The listing builds one solid part. Answer for the finished solid, in the listing's coordinates (mm). Give positions to 0.01 mm unless a question says otherwise; leave off trailing zeros. Order: outer loops, then holes, each group sorted by start corner. A loop starts at its lowest first (then second) coordinate and runs counter-clockwise, first axis right, second up. Notation, with made-up numbers: (-33.75, 8) - (12.25, 8) arc R32 cw to (12.25, 35) - close; hole circle Ø5 at (32.25, 65.5). An arc over 180 degrees is marked (long way). Answer as a JSON object with one key per item and string values. Group by question number.
Q1. A cutting plane is placed at B-B, the plane y = 4. Give the vertices of the cut face in (x, z), and give its area (3 significant figures).
Q2. Consider line 1 (Y direction, x = -5.5, z = 304.5); line 2 (Y direction, x = -13, z = 213.5). Determine where each line is inside the solid, lowest interval first.
Q3. A cutting plane is placed at C-C, the plane z = 54. Give the vertices of the cut face in (x, y).
Q4. A cutting plane is placed at A-A, the plane x = -6. Give the vertices of the cut face in (y, z).
Q5. Given pin 1 (2 mm diameter, centred on x = 6, y = -12.5, fed in from +Z), flat-ended and moving along its own axis, determine where the tip first touches the part or whether it passes through.
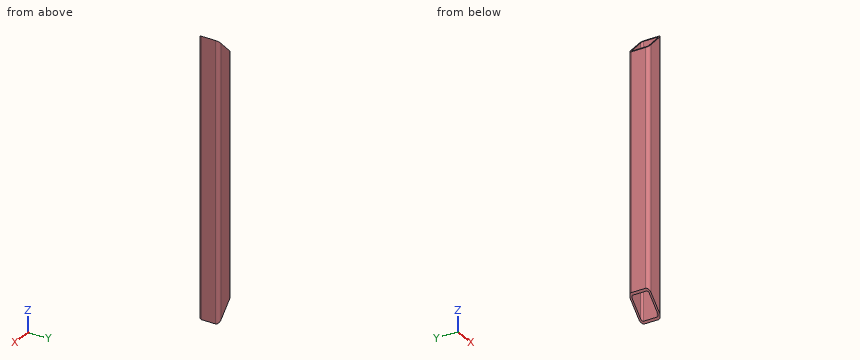
Autodesk Inventor part; units mm, degrees
ref_plane "Start plane" through (0, 0, -17.5) normal (0, 0, 1) x (1, 0, 0)
ref_plane "End plane" through (0, 0, 447.5) normal (0, 0, 1) x (1, 0, 0)
ref_plane "Work Plane5" through (17.5, 0, 447.5) normal (-0.7071, 0, 0.7071) x (0.7071, 0, 0.7071)
ref_plane "Start plane" through (0, 0, -17.5) normal (0, 0, 1) x (1, 0, 0)
ref_plane "End plane" through (0, 0, 447.5) normal (0, 0, 1) x (1, 0, 0)
sketch "Sketch" plane through (0, 0, 0) normal (0, 0, 1) x (1, 0, 0)
  line L0 (-17.5, -11.5) -> (-17.5, 11.5)
  line L1 (-11.5, 17.5) -> (11.5, 17.5)
  line L2 (17.5, 11.5) -> (17.5, -11.5)
  line L3 (11.5, -17.5) -> (-11.5, -17.5)
  arc A0 (-17.5, -11.5) -> (-11.5, -17.5) centre (-11.5, -11.5) ccw
  arc A1 (-11.5, 17.5) -> (-17.5, 11.5) centre (-11.5, 11.5) ccw
  arc A2 (17.5, 11.5) -> (11.5, 17.5) centre (11.5, 11.5) ccw
  arc A3 (11.5, -17.5) -> (17.5, -11.5) centre (11.5, -11.5) ccw
  arc A4 (-11.5, 14.5) -> (-14.5, 11.5) centre (-11.5, 11.5) ccw
  line L4 (-11.5, 14.5) -> (11.5, 14.5)
  arc A5 (14.5, 11.5) -> (11.5, 14.5) centre (11.5, 11.5) ccw
  line L5 (14.5, 11.5) -> (14.5, -11.5)
  arc A6 (11.5, -14.5) -> (14.5, -11.5) centre (11.5, -11.5) ccw
  line L6 (11.5, -14.5) -> (-11.5, -14.5)
  arc A7 (-14.5, -11.5) -> (-11.5, -14.5) centre (-11.5, -11.5) ccw
  line L7 (-14.5, -11.5) -> (-14.5, 11.5)
  line L8 (0, 25.4278) -> (0, -25.4278) construction
  line L9 (-25.4278, 0) -> (25.4278, 0) construction
  dimension "d7" = 6
  dimension "d10" = 35
  dimension "d11" = 35
  dimension "d12" = 3
  dimension "d15" = 17.5
  dimension "d16" = 17.5
extrude "Body" add sketch "Sketch" along normal up to surface (465 mm away) from surface at -17.5
sketch "Sketch3" plane through (0, 0, 0) normal (0, 0, 1) x (1, 0, 0)
  line L0 (0, 0) -> (10, 0)
ref_plane "Work Plane3" through (0, 0, 0) normal (0, -1, 0) x (1, 0, 0)
sketch "Sketch4" plane through (0, 0, 0) normal (0, -1, 0) x (1, 0, 0)
  line L0 (-2, -17.5) -> (12, -17.5)
  line L1 (-2, 447.5) -> (12, 447.5)
  dimension "d18" = 465
ref_plane "Work Plane5" through (17.5, 0, 447.5) normal (-0.7071, 0, 0.7071) x (0.7071, 0, 0.7071)
split "Split2" plane through (17.5, 0, 447.5) removes the side toward (-0.7071, 0, 0.7071)
ref_plane "Work Plane12" through (0, 180, -17.5) normal (0, 0, -1) x (-1, 0, 0)
split "Split6" plane through (0, 180, -17.5) removes the side toward (0, 0, -1)
ref_plane "Work Plane13" through (17.5, 0, -17.5) normal (-0.7071, 0, -0.7071) x (-0.7071, 0, 0.7071)
split "Split7" plane through (17.5, 0, -17.5) removes the side toward (-0.7071, 0, -0.7071)
equation "\"d7\" = G_IR"
equation "\"d10\" = G_H"
equation "\"d11\" = G_W"
equation "\"d12\" = G_T"
equation "\"d15\" = 0.5 * d10"
equation "\"d16\" = 0.5 * d11"
equation "\"d3\" = G_L"
equation "\"G_W\" = 35"
equation "\"G_H\" = 35"
equation "\"G_T\" = 3"
equation "\"G_IR\" = 6"
equation "\"G_L\" = d18"
equation "\"G_OFFSET_START\" = 17.5"
equation "\"G_OFFSET_END\" = 17.5"
equation "\"d13\" = -G_OFFSET_START"
equation "\"d14\" = G_OFFSET_END + B_L"
properties part number "AS 1163 - C350L0 35x35x3.0 SHS - 465" material "Steel, Mild"
Reply:
{
 "1": {"outline": "(-17.5, 17.5) - (-14.5, 14.5) - (-14.5, 415.5) - (-17.5, 412.5) - close; (14.5, -14.5) - (17.5, -17.5) - (17.5, 447.5) - (14.5, 444.5) - close", "area": "2,580 mm^2"},
 "2": {"line 1": "y = -17.5 to -14.5, 14.5 to 17.5", "line 2": "y = -17.31 to -14.1, 14.1 to 17.31"},
 "3": {"outline": "(-17.5, -11.5) arc R6 ccw to (-11.5, -17.5) - (11.5, -17.5) arc R6 ccw to (17.5, -11.5) - (17.5, 11.5) arc R6 ccw to (11.5, 17.5) - (-11.5, 17.5) arc R6 ccw to (-17.5, 11.5) - close; hole (-14.5, -11.5) arc R3 ccw to (-11.5, -14.5) - (11.5, -14.5) arc R3 ccw to (14.5, -11.5) - (14.5, 11.5) arc R3 ccw to (11.5, 14.5) - (-11.5, 14.5) arc R3 ccw to (-14.5, 11.5) - close"},
 "4": {"outline": "(-17.5, 6) - (-14.5, 6) - (-14.5, 424) - (-17.5, 424) - close; (14.5, 6) - (17.5, 6) - (17.5, 424) - (14.5, 424) - close"},
 "5": {"pin 1": "passes through"}
}
